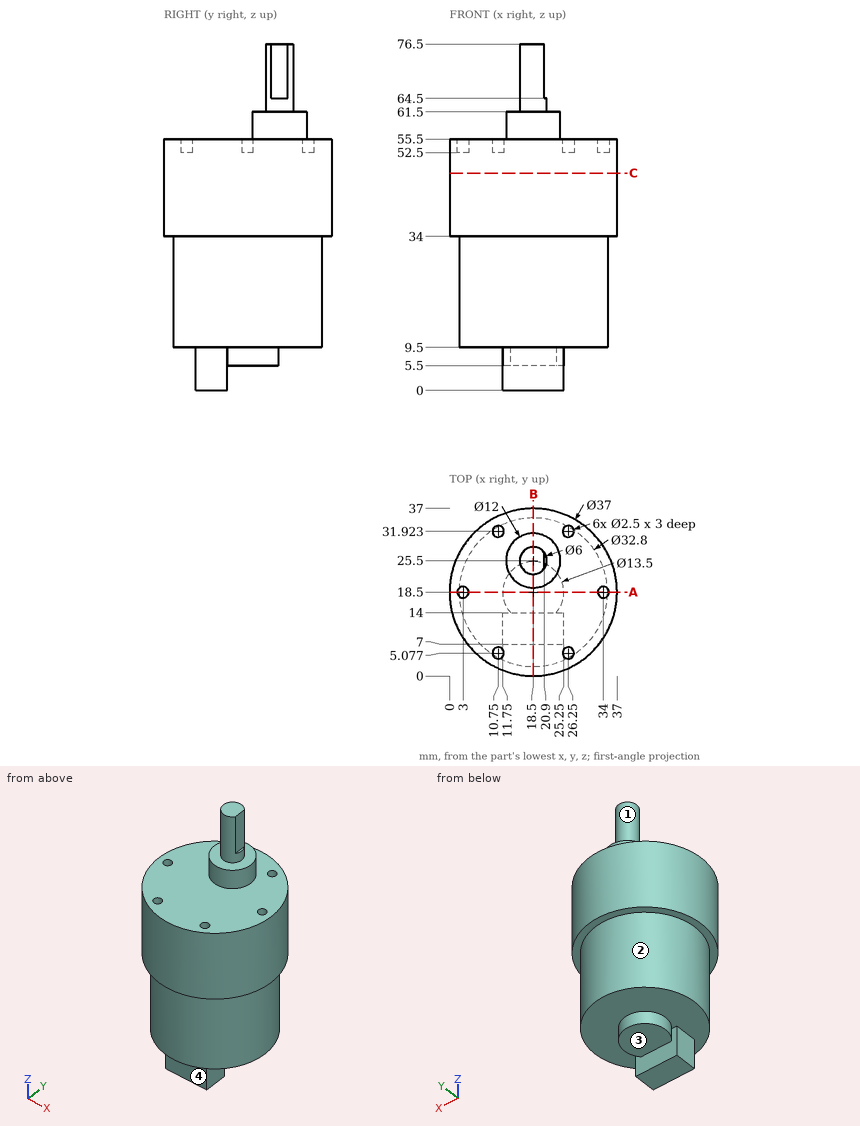
Study the drawing (mm; zero at the part's minimum x, y, z) and answer. A direction names the side the tool comes from. Give positions to 0.01 mm unless a question says otherwise; leave off trailing zeros. Write each loop counter-clockwise with the first axis right and the second up, starting at its lowest first coordinate (ties: lowest second). Pieces come first, ordered by that corner, then holes. Notation, with made-up numbers: M -20.5,45 L 24.5,45 A21 ccw 24.5,67 Z; hole C 62,-4.75 d1. An arc over 180 degrees is marked long. Put each result on its own line as item: value. Start each with the question number.
1. Each of these flat-tipped pins is pushed along its axis until it touches: pin 1 Ø6 at (y, z) = (18.5, 63) entering from -X; pin 2 Ø3 at (y, z) = (26.5, 54) entering from +X; pin 3 Ø2 at (x, y) = (26.25, 5.08) entering from -Z. Where does it stop, or does it pass through?
2. Which of the six approach directions +Z, -Z, +X, -X, +Y, -Y give full straight-line access (tool end or side, diameter ignored) to the marked faces 1, 2, 3 and 4?
3. The part is cut by section C-C, the plane z = 48. Give the vertices of the cut face in (x, y).
4. The part is cut by section B-B, the plane x = 18.5. Give the vertices of the cut face in (y, z), and give its area (3 significant figures).
5. Consider line 1 along Y through (x, z) = (10.75, 53.85); line 2 along Z through (x, y) = (19, 31); line 3 along Z through (x, y) = (32.5, 15.5). Determine where each line is inside the solid, lowest interval first.
6. The part is cut by section A-A, the plane y = 18.5. Give the vertices of the cut face in (x, z).
Final values:
1. pin 1: stops at x = 14.42
1. pin 2: stops at x = 35.82
1. pin 3: stops at z = 9.5
2. face 1: +Z
2. face 2: -Z
2. face 3: -Z, +X, -X, +Y
2. face 4: -Z, +X, -X, -Y
3. outline: C 18.5,18.5 d37
4. outline: M 0,34 L 2.1,34 L 2.1,9.5 L 7,9.5 L 7,0 L 14,0 L 14,5.5 L 25.25,5.5 L 25.25,9.5 L 34.9,9.5 L 34.9,34 L 37,34 L 37,55.5 L 31.5,55.5 L 31.5,61.5 L 28.5,61.5 L 28.5,76.5 L 22.5,76.5 L 22.5,61.5 L 19.5,61.5 L 19.5,55.5 L 0,55.5 Z
4. area: 1,870 mm²
5. line 1: y = 1.7 to 3.83, 6.33 to 30.67, 33.17 to 35.3
5. line 2: z = 9.5 to 61.5
5. line 3: z = 9.5 to 55.5
6. outline: M 0,34 L 2.1,34 L 2.1,9.5 L 11.75,9.5 L 11.75,5.5 L 25.25,5.5 L 25.25,9.5 L 34.9,9.5 L 34.9,34 L 37,34 L 37,55.5 L 35.25,55.5 L 35.25,52.5 L 32.75,52.5 L 32.75,55.5 L 4.25,55.5 L 4.25,52.5 L 1.75,52.5 L 1.75,55.5 L 0,55.5 Z
